```python
from build123d import *

# Parameters (mm, degrees)
SKETCH1_R                    = 5
BOSS_EXTRUDE1_DEPTH          = 30
SKETCH2_R                    = 30
BOSS_EXTRUDE2_DEPTH          = 20
BOSS_EXTRUDE3_DEPTH          = 10
BOSS_EXTRUDE4_DEPTH          = 60
CUT_EXTRUDE2_DEPTH           = 107.979678493
SCHIZZO1_W                   = 77.430619172
SCHIZZO1_H                   = 31.885326398
ESTRUSIONE_ESTRUSIONE1_DEPTH = 220
SKETCH8_R                    = 15
CUT_EXTRUDE3_DEPTH           = 10
SKETCH9_R                    = 20
CUT_EXTRUDE4_DEPTH           = 10


with BuildPart() as part:
    # Sketch1 → Boss-Extrude1 (new, symmetric)
    with BuildSketch(Plane.XY):
        Circle(SKETCH1_R)
    extrude(amount=BOSS_EXTRUDE1_DEPTH, both=True)

    # Sketch2 → Boss-Extrude2 (add)
    with BuildSketch(Plane.XY.offset(30)):
        Circle(SKETCH2_R)
    boss_extrude2 = extrude(amount=BOSS_EXTRUDE2_DEPTH)

    # Mirror1: Boss-Extrude2 across plane
    add(boss_extrude2.mirror(Plane.XY))

    # Sketch5 → Boss-Extrude3 (add)
    with BuildSketch(Plane.XY.offset(50)):
        with BuildLine():
            Line((49.046850524, 30), (49.046850524, -30))
            Line((49.046850524, -30), (0, -30))
            ThreePointArc((0, -30), (-30, 0), (0, 30))
            Line((0, 30), (49.046850524, 30))
        make_face()
    boss_extrude3 = extrude(amount=BOSS_EXTRUDE3_DEPTH)

    # Mirror3: Boss-Extrude3 across plane
    add(boss_extrude3.mirror(Plane.XY))

    # Sketch6 → Boss-Extrude4 (add, symmetric)
    with BuildSketch(Plane.XY):
        Polygon((49.046850524, -30), (49.046850524, 30), (83.33457632, 15.942663199), (83.33457632, -15.942663199), align=None)
    extrude(amount=BOSS_EXTRUDE4_DEPTH, both=True)

    # Sketch7 → Cut-Extrude2 (cut, symmetric)
    with BuildSketch(Plane(origin=(0, 0, 0), x_dir=(1, 0, 0), z_dir=(0, 1, 0))):
        Polygon((-220.635461706, 227.409893565), (49.046850524, 60), (92.240822161, 33.186605623), (361.923134392, -134.223287942), (696.742921522, 405.141336519), (114.184325424, 766.774518026), align=None)
    cut_extrude2 = extrude(amount=CUT_EXTRUDE2_DEPTH, both=True, mode=Mode.SUBTRACT)

    # Mirror4: Cut-Extrude2 across plane
    add(cut_extrude2.mirror(Plane.XY), mode=Mode.SUBTRACT)

    # Schizzo1 → Estrusione-Estrusione1 (add)
    with BuildSketch(Plane(origin=(83.33457632, 0, 0), x_dir=(0, 0, -1), z_dir=(1, 0, 0))):
        Rectangle(SCHIZZO1_W, SCHIZZO1_H)
    extrude(amount=ESTRUSIONE_ESTRUSIONE1_DEPTH)

    # Sketch8 → Cut-Extrude3 (cut)
    with BuildSketch(Plane(origin=(303.33457632, 0, 0), x_dir=(0, 0, -1), z_dir=(1, 0, 0))):
        Circle(SKETCH8_R)
    extrude(amount=-CUT_EXTRUDE3_DEPTH, mode=Mode.SUBTRACT)

    # Sketch9 → Cut-Extrude4 (cut)
    with BuildSketch(Plane(origin=(293.33457632, 0, 0), x_dir=(0, 0, -1), z_dir=(1, 0, 0))):
        Circle(SKETCH9_R)
    extrude(amount=-CUT_EXTRUDE4_DEPTH, mode=Mode.SUBTRACT)


solid = part.part
```
Source: CAD feature listing. Evaluate the final solid. Frame: model axes, mm. A direction names the side the tool comes from. Round coordinates to 2 decimals unless told otherwise and drop trailing zeros. Write each loop counter-clockwise with the first axis right and the second up, starting at its lowest first coordinate (ties: lowest second). Pieces come first, ordered by that corner, then holes. Notation, with made-up numbers: M 2.25,50 L 40.25,50 A19 cw 40.25,66 Z; hole C -22.5,61 d3. An arc over 180 degrees is marked long. Answer as a JSON object with one key per item and string values. Group by question number.
(1) Section query A-A on y = 0. Output: boundary loops of the cut face in (x, z).
(2) Reachability of faces 4 (the flat face through (25, -30, -55)), 5 (the flat face through (65.95, 23.07, 0.84)), 6 (the flat face through (293.335, 10, 12)), 7 (the flat face through (192, -15.943, 1)), 8 (the flat face through (49.047, 0, 1)) from +Z, -Z, +X, -X, +Y, -Y: full face, straight path, thin tool, end or side. Return the list, or none.
(3) Mould query, pull axis Z, two halves, no side actions, for faces 1 (the flat face through (36, 0, 50)), 2 (the flat face through (66.431, -22.873, 0.84)), 3 (the flat face through (192, 0, -38.715)). Classes: +Z half, -Z half, draft (parallel to the pull), parting line (faces both ways), or undercut.
(4) Ray query, line 1 (Y direction, x = 300, z = 0); line 2 (Z direction, x = 3.5, y = -11); line 3 (Z direction, x = 45, y = -5). Return the intervals inside material, ascending. Write a range as [from, to].
(5) First-contact query: pin 1 (4 mm diameter, centred on x = 120, z = 20, fed in from +Y); pin 2 (12 mm diameter, centred on y = -15.5, z = -16.5, fed in from -X); pin 3 (16 mm diameter, centred on x = 160, y = 5.5, fed in from +Z). Flat tips, straight axial feed; report the tip coordinate or a pass-through.
Computed values:
{
 "1": {"outline": "M -30,-60 L 49.05,-60 L 83.33,-38.72 L 303.33,-38.72 L 303.33,-15 L 293.33,-15 L 293.33,-20 L 283.33,-20 L 283.33,20 L 293.33,20 L 293.33,15 L 303.33,15 L 303.33,38.72 L 83.33,38.72 L 49.05,60 L -30,60 L -30,30 L -5,30 L -5,-30 L -30,-30 Z; hole M 5,-30 L 30,-30 L 30,-50 L 49.05,-50 L 49.05,50 L 30,50 L 30,30 L 5,30 Z"},
 "2": {"face 4": "+Z, -Z, +X, -X, -Y", "face 5": "+Z, -Z, +X, +Y", "face 6": "none", "face 7": "+Z, -Z, +X, -Y", "face 8": "+Y, -Y"},
 "3": {"face 1": "undercut", "face 2": "draft", "face 3": "-Z half"},
 "4": {"line 1": "[-15.94, -15], [15, 15.94]", "line 2": "[-60, -30], [30, 60]", "line 3": "[-60, -50], [50, 60]"},
 "5": {"pin 1": "y = 15.94", "pin 2": "x = 49.05", "pin 3": "z = 38.72"}
}
